Autodesk Inventor part; units mm, degrees
ref_plane "YZ Plane" through (0, 0, 0) normal (1, 0, 0) x (0, 1, 0)
ref_plane "XZ Plane" through (0, 0, 0) normal (0, 1, 0) x (-1, 0, 0)
ref_plane "XY Plane" through (0, 0, 0) normal (0, 0, 1) x (1, 0, 0)
sketch "스케치1" plane through (0, 0, 0) normal (0, 0, 1) x (1, 0, 0)
  line L0 (-21.75, -10) -> (21.75, -10)
  line L1 (21.75, -10) -> (21.75, 10)
  line L2 (21.75, 10) -> (-21.75, 10)
  line L3 (-21.75, 10) -> (-21.75, -10)
  line L4 (-21.75, -10) -> (21.75, 10) construction
  line L5 (21.75, -10) -> (-21.75, 10) construction
  circle A0 centre (-14.75, -7.5) radius 1.25
  circle A1 centre (3.25, -7.5) radius 1.25
  circle A2 centre (-14.75, 7.5) radius 1.25
  circle A3 centre (3.25, 7.5) radius 1.25
  point P0 (0, 0)
  dimension "d0" = 43.5
  dimension "d1" = 20
  dimension "d4" = 2.5
  dimension "d5" = 2.5
  dimension "d6" = 7
  dimension "d9" = 18
  dimension "d12" = 15
extrude "돌출1" add sketch "스케치1" along normal blind 6
properties part number "dc_convertor" material "고무, 검은색"
Design review of the part built by this model. Coordinates are the model's own, in mm. Round coordinates to 2 decimals unless told otherwise and drop trailing zeros. Write each loop counter-clockwise with the first axis right and the second up, starting at its lowest first coordinate (ties: lowest second). Pieces come first, ordered by that corner, then holes. Notation, with made-up numbers: (-39, 24.5) - (14, 24.5) arc R17 ccw to (14, 52.5) - close; hole circle Ø5 at (7, 61.25). An arc over 180 degrees is marked (long way). Return JSON: item names as keys, results as strings. Group by question number.
Item 1: For probe 1 along Y at (x, z) = (-14.75, 2.1); probe 2 along Y at (x, z) = (4, 2.65); probe 3 along X at (y, z) = (7, 5.05), list the stretches that pass through material, from the lowest coordinate up. Write a range as [from, to].
Item 2: We need section B-B on z = 4.75. Write out the cut boundary in (x, y), and give its area (3 significant figures).
Item 3: We need section C-C on x = 3.25. Write out the cut boundary in (y, z), and give its area (3 significant figures).
Item 4: We need section A-A on y = 7.5. Write out the cut boundary in (x, z).
Item 5: The part is to be moulded in two halves that separate along Y. For faces 1 (the face through (0, 0, 0)), 2 (the face through (-15.74, -6.74, 2.96)), 3 (the face through (4.405, 7.979, 2.958)), 4 (the face through (0, 10, 3)), say which applies: pulls with the +Y half, pulls with the -Y half, needs draft (parallel to the pull), parting line crosses it, or undercut.
Model answer:
{
 "1": {"probe 1": "y = [-10, -8.75], [-6.25, 6.25], [8.75, 10]", "probe 2": "y = [-10, -8.5], [-6.5, 6.5], [8.5, 10]", "probe 3": "x = [-21.75, -15.9], [-13.6, 2.1], [4.4, 21.75]"},
 "2": {"outline": "(-21.75, -10) - (21.75, -10) - (21.75, 10) - (-21.75, 10) - close; hole circle Ø2.5 at (-14.75, -7.5); hole circle Ø2.5 at (-14.75, 7.5); hole circle Ø2.5 at (3.25, -7.5); hole circle Ø2.5 at (3.25, 7.5)", "area": "850 mm²"},
 "3": {"outline": "(-10, 0) - (-8.75, 0) - (-8.75, 6) - (-10, 6) - close; (-6.25, 0) - (6.25, 0) - (6.25, 6) - (-6.25, 6) - close; (8.75, 0) - (10, 0) - (10, 6) - (8.75, 6) - close", "area": "90.0 mm²"},
 "4": {"outline": "(-21.75, 0) - (-16, 0) - (-16, 6) - (-21.75, 6) - close; (-13.5, 0) - (2, 0) - (2, 6) - (-13.5, 6) - close; (4.5, 0) - (21.75, 0) - (21.75, 6) - (4.5, 6) - close"},
 "5": {"face 1": "needs draft", "face 2": "undercut", "face 3": "undercut", "face 4": "pulls with the +Y half"}
}
